Part model, mm, in its own coordinate system. A direction names the side the tool comes from. Coordinates: 2 decimals unless noted, no trailing zeros. Loops run counter-clockwise (first coordinate to the right, second up) from the corner with the lowest first, then second, coordinate; pieces in that order, holes last. Notation, with made-up numbers: (-13, -6) -> (17, -6) arc R23 cw to (17, 11) -> close; hole circle Ø5 at (24.25, 31.5). An arc over 180 degrees is marked (long way). One line per question, with ' | ' between items. Start each with the question number.
1) Cut at D-D (y = 2.5). Count the separate pieces of the cut face and the enclosed holes in it, plus the area to 3 significant figures.
2) Cut at C-C (x = 3.25). List the corners of the cut face in (y, z) (3 decimals), plus the area to 4 significant figures.
3) Cut at B-B (z = 1). List the corners of the cut face in (x, y) (3 decimals).
4) Two-plate mould, pull along X, no slides. Class faces 1 (the face through (-3, 2, -2.27)), 2 (the face through (2, -5, -0.725)), 3 (the face through (-6.125, -1, 0)): released by +X, released by -X, zero draft, split by the parting line, or undercut.
5) Drop flat-ended pins along their axis: pin 1 (1.2 mm diameter, centred on x = -3, y = -5, fed in from +Z) (3 decimals); pin 2 (0.6 mm diameter, centred on x = 2.5, z = 1.5, fed in from +Y); pin 3 (1.2 mm diameter, centred on x = 2, y = -4.5, fed in from -Z) (3 decimals). Give the stop position or say it passes through.
6) Cut at A-A (y = -4.25). List the corners of the cut face in (x, z) (3 decimals).
7) 3-axis set-ups, long thin cutter, end or side, ignore diameter. For faces 4 (the face through (1.9, -0.7, -3.5)), 5 (the face through (-1, 2, 1)), 6 (the face through (-1.9, -0.6, -3.5)), 7 (the face through (-3, -5, -0.725)): which of +Z, -Z, +X, -X, +Y, -Y reach the whole face in a straight line?
8) Probe L1, parallel to Z at x = -2.25, y = 1.5; L2, parallel to X at y = -5, z = -0.5 (3 decimals); L3, parallel to X at y = -0.25, z = -3.25. List the from-to ranges inside material, lowest first. Write a range as from..to.
from build123d import *

# Parameters (mm, degrees)
EXTRUDE_1_DEPTH     = 3
EXTRUDE_START       = -4
EXTRUDE_2_DEPTH     = 1
SKETCH_2_W          = 2
SKETCH_2_H          = 2
CUT_EXTRUDE_1_DEPTH = 3
SKETCH_3_W          = 1.5
SKETCH_3_H          = 0.3
EXTRUDE_3_DEPTH     = 2.5


with BuildPart() as part:
    # Эскиз1 → Бобышка-Вытянуть1 (new, symmetric)
    with BuildSketch(Plane.XY):
        Polygon((-6.125, 1.5), (-6.125, -3.5), (-1.9, -3.5), (-1.9, 2.122094745), (-1.129392625, 2.998992793), (1.129392625, 2.998992793), (1.9, 2.122094745), (1.9, -3.5), (6.125, -3.5), (6.125, 1.5), (5, 3.5), (-5, 3.5), align=None)
        Polygon((-1.9, 2.122094745), (-1.9, -3.5), (1.9, -3.5), (1.9, 2.122094745), (1.129392625, 2.998992793), (-1.129392625, 2.998992793), align=None)
    extrude(amount=EXTRUDE_1_DEPTH, both=True)

    # Эскиз1<3> → Бобышка-Вытянуть2 (add)
    with BuildSketch(Plane.XY.offset(EXTRUDE_START)):
        Polygon((-1.9, 2.122094745), (-1.9, -3.5), (1.9, -3.5), (1.9, 2.122094745), (1.129392625, 2.998992793), (-1.129392625, 2.998992793), align=None)
    extrude(amount=EXTRUDE_2_DEPTH)

    # Эскиз2 → Вырез-Вытянуть1 (cut)
    with BuildSketch(Plane(origin=(0, 3.5, 0), x_dir=(1, 0, 0), z_dir=(0, 1, 0))):
        with Locations((0, 1.27)):
            Rectangle(SKETCH_2_W, SKETCH_2_H)
        with Locations((0, -1.27)):
            Rectangle(SKETCH_2_W, SKETCH_2_H)
        with Locations((2.54, 1.27)):
            Rectangle(SKETCH_2_W, SKETCH_2_H)
        with Locations((2.54, -1.27)):
            Rectangle(SKETCH_2_W, SKETCH_2_H)
        with Locations((-2.54, 1.27)):
            Rectangle(SKETCH_2_W, SKETCH_2_H)
        with Locations((-2.54, -1.27)):
            Rectangle(SKETCH_2_W, SKETCH_2_H)
    extrude(amount=-CUT_EXTRUDE_1_DEPTH, mode=Mode.SUBTRACT)

    # Эскиз3 → Бобышка-Вытянуть3 (add)
    with BuildSketch(Plane.XZ.offset(3.5)):
        with Locations((-3.175, -0.575)):
            Rectangle(SKETCH_3_W, SKETCH_3_H)
        with Locations((-1.905, 0.575)):
            Rectangle(SKETCH_3_W, SKETCH_3_H)
        with Locations((-0.635, -0.575)):
            Rectangle(SKETCH_3_W, SKETCH_3_H)
        with Locations((0.635, 0.575)):
            Rectangle(SKETCH_3_W, SKETCH_3_H)
        with Locations((1.905, -0.575)):
            Rectangle(SKETCH_3_W, SKETCH_3_H)
        with Locations((3.175, 0.575)):
            Rectangle(SKETCH_3_W, SKETCH_3_H)
    extrude(amount=EXTRUDE_3_DEPTH)


solid = part.part
Reported:
1) separate pieces: 1 | enclosed holes: 6 | area: 45.9 mm²
2) outline: (-6, 0.425) -> (-3.5, 0.425) -> (-3.5, -3) -> (3.5, -3) -> (3.5, -2.27) -> (0.5, -2.27) -> (0.5, -0.27) -> (3.5, -0.27) -> (3.5, 0.27) -> (0.5, 0.27) -> (0.5, 2.27) -> (3.5, 2.27) -> (3.5, 3) -> (-3.5, 3) -> (-3.5, 0.725) -> (-6, 0.725) -> close | area: 30.75 mm²
3) outline: (-6.125, -3.5) -> (6.125, -3.5) -> (6.125, 1.5) -> (5, 3.5) -> (3.54, 3.5) -> (3.54, 0.5) -> (1.54, 0.5) -> (1.54, 3.5) -> (1, 3.5) -> (1, 0.5) -> (-1, 0.5) -> (-1, 3.5) -> (-1.54, 3.5) -> (-1.54, 0.5) -> (-3.54, 0.5) -> (-3.54, 3.5) -> (-5, 3.5) -> (-6.125, 1.5) -> close
4) face 1: undercut | face 2: zero draft | face 3: released by -X
5) pin 1: stops at z = 0.725 | pin 2: stops at y = 0.5 | pin 3: stops at z = -0.725
6) outline: (-3.925, -0.725) -> (-2.425, -0.725) -> (-2.425, -0.425) -> (-3.925, -0.425) -> close; (-2.655, 0.425) -> (-1.155, 0.425) -> (-1.155, 0.725) -> (-2.655, 0.725) -> close; (-1.385, -0.725) -> (0.115, -0.725) -> (0.115, -0.425) -> (-1.385, -0.425) -> close; (-0.115, 0.425) -> (1.385, 0.425) -> (1.385, 0.725) -> (-0.115, 0.725) -> close; (1.155, -0.725) -> (2.655, -0.725) -> (2.655, -0.425) -> (1.155, -0.425) -> close; (2.425, 0.425) -> (3.925, 0.425) -> (3.925, 0.725) -> (2.425, 0.725) -> close
7) face 4: -Z, +X, +Y, -Y | face 5: +Y | face 6: -Z, -X, +Y, -Y | face 7: -Z, +X, -X, -Y
8) L1: z = -3..-2.27, -0.27..0.27, 2.27..3 | L2: x = -3.925..-2.425, -1.385..0.115, 1.155..2.655 | L3: x = -1.9..1.9
